from build123d import *

# Parameters (mm, degrees)
BASE_FLANGE1_DEPTH           = 2.65684
EDGE_FLANGE1_DEPTH           = 254
EDGE_FLANGE2_STRIP_W         = 16.97736
EDGE_FLANGE2_STRIP_H         = 2.65684
EDGE_FLANGE2_STRIP_CUT_DEPTH = 112.395
EDGE_FLANGE2_DEPTH           = 112.395
EDGE_FLANGE3_DEPTH           = 112.395
EDGE_FLANGE4_DEPTH           = 248.16816
SKETCH22_R                   = 6.35
CUT_EXTRUDE1_DEPTH           = 2.65684
SKETCH23_R                   = 6.35
CUT_EXTRUDE2_DEPTH           = 2.65684
SKETCH24_R                   = 6.35
CUT_EXTRUDE3_DEPTH           = 2.65684


# Sheet-metal steps are written as plain solids
with BuildPart() as part:
    # Sketch1 → Base-Flange1 (new body)
    with BuildSketch(Plane.XY):
        with BuildLine():
            Line((0, 0), (355.6, 0))
            Line((355.6, 0), (355.6, 254))
            Line((355.6, 254), (193.04, 254))
            ThreePointArc((193.04, 254), (177.8, 238.76), (162.56, 254))
            Line((162.56, 254), (0, 254))
            Line((0, 254), (0, 0))
        make_face()
    extrude(amount=-BASE_FLANGE1_DEPTH)

    # Edge-Flange1 section (across the edge) → Edge-Flange1 (add)
    with BuildSketch(Plane(origin=(-3.175, 0, -2.65684), x_dir=(1, 0, 0), z_dir=(0, 1, 0))):
        with BuildLine():
            Line((-2.65684, 3.175), (-2.65684, 115.57))
            Line((-2.65684, 115.57), (0, 115.57))
            Line((0, 115.57), (0, 3.175))
            ThreePointArc((0, 3.175), (0.92993597, 0.92993597), (3.175, 0))
            Line((3.175, 0), (3.175, -2.65684))
            ThreePointArc((3.175, -2.65684), (-0.948733611, -0.948733611), (-2.65684, 3.175))
        make_face()
    extrude(amount=EDGE_FLANGE1_DEPTH)

    # Edge-Flange2 strip (across the edge) → Edge-Flange2 strip cut (cut)
    with BuildSketch(Plane(origin=(-5.83184, 254, -5.83184), x_dir=(0, -1, 0), z_dir=(0, 0, -1))):
        with Locations((-2.65684, -1.32842)):
            Rectangle(EDGE_FLANGE2_STRIP_W, EDGE_FLANGE2_STRIP_H)
    extrude(amount=EDGE_FLANGE2_STRIP_CUT_DEPTH, mode=Mode.SUBTRACT)

    # Edge-Flange2 section (across the edge) → Edge-Flange2 (add)
    with BuildSketch(Plane(origin=(-5.83184, 254, -5.83184), x_dir=(0, -1, 0), z_dir=(0, 0, -1))):
        with BuildLine():
            Line((0, 3.175), (0, 57.15))
            Line((0, 57.15), (2.65684, 57.15))
            Line((2.65684, 57.15), (2.65684, 3.175))
            ThreePointArc((2.65684, 3.175), (3.58677597, 0.92993597), (5.83184, 0))
            Line((5.83184, 0), (5.83184, -2.65684))
            ThreePointArc((5.83184, -2.65684), (1.708106389, -0.948733611), (0, 3.175))
        make_face()
    extrude(amount=EDGE_FLANGE2_DEPTH)

    # Edge-Flange3 section (across the edge) → Edge-Flange3 (add)
    with BuildSketch(Plane(origin=(-5.83184, -3.175, -118.22684), x_dir=(0, 1, 0), z_dir=(0, 0, 1))):
        with BuildLine():
            Line((-2.65684, 3.175), (-2.65684, 57.15))
            Line((-2.65684, 57.15), (0, 57.15))
            Line((0, 57.15), (0, 3.175))
            ThreePointArc((0, 3.175), (0.92993597, 0.92993597), (3.175, 0))
            Line((3.175, 0), (3.175, -2.65684))
            ThreePointArc((3.175, -2.65684), (-0.948733611, -0.948733611), (-2.65684, 3.175))
        make_face()
    extrude(amount=EDGE_FLANGE3_DEPTH)

    # Edge-Flange4 section (across the edge) → Edge-Flange4 (add)
    with BuildSketch(Plane(origin=(-3.175, 0, -121.40184), x_dir=(0, 0, 1), z_dir=(0, 1, 0))):
        with BuildLine():
            Line((-2.65684, 3.175), (-2.65684, 25.4))
            Line((-2.65684, 25.4), (0, 25.4))
            Line((0, 25.4), (0, 3.175))
            ThreePointArc((0, 3.175), (0.92993597, 0.92993597), (3.175, 0))
            Line((3.175, 0), (3.175, -2.65684))
            ThreePointArc((3.175, -2.65684), (-0.948733611, -0.948733611), (-2.65684, 3.175))
        make_face()
    extrude(amount=EDGE_FLANGE4_DEPTH)

    # Sketch22 → Cut-Extrude1 (cut)
    with BuildSketch(Plane(origin=(0, 254, 0), x_dir=(1, 0, 0), z_dir=(0, 1, 0))):
        with Locations(Location((-40.76446, 86.995, 0), (0, 0, 180))):
            Circle(SKETCH22_R)
        with Locations(Location((-40.76446, 36.195, 0), (0, 0, 180))):
            Circle(SKETCH22_R)
    extrude(amount=-CUT_EXTRUDE1_DEPTH, mode=Mode.SUBTRACT)

    # Sketch23 → Cut-Extrude2 (cut)
    with BuildSketch(Plane(origin=(0, -3.175, 0), x_dir=(1, 0, 0), z_dir=(0, 1, 0))):
        with Locations(Location((-34.40684, 86.36, 0), (0, 0, 180))):
            Circle(SKETCH23_R)
        with Locations(Location((-34.40684, 35.56, 0), (0, 0, 180))):
            Circle(SKETCH23_R)
    extrude(amount=-CUT_EXTRUDE2_DEPTH, mode=Mode.SUBTRACT)

    # Sketch24 → Cut-Extrude3 (cut)
    with BuildSketch(Plane.ZY.offset(5.83184)):
        with Locations((-86.995, 41.79316)):
            Circle(SKETCH24_R)
        with Locations((-34.40684, 41.79316)):
            Circle(SKETCH24_R)
    extrude(amount=-CUT_EXTRUDE3_DEPTH, mode=Mode.SUBTRACT)


solid = part.part
For this review, take the finished solid that the model builds, in its own axes (mm). A direction names the side the tool comes from. Round coordinates to 2 decimals unless told otherwise and drop trailing zeros. Write each loop counter-clockwise with the first axis right and the second up, starting at its lowest first coordinate (ties: lowest second). Pieces come first, ordered by that corner, then holes. Notation, with made-up numbers: (25, 27.25) -> (32, 27.25) arc R15 ccw to (32, 51.25) -> close; hole circle Ø11 at (63, 67.5). An arc over 180 degrees is marked (long way). Put each result on its own line as item: value.
Q1. Consider section B-B on z = -70.5. State the section outline as (x, y) points (3 decimals), and give its area (3 significant figures).
Determined:
outline: (-62.982, -5.832) -> (-9.007, -5.832) arc R5.832 ccw to (-3.175, 0) -> (-3.175, 248.168) arc R5.832 ccw to (-9.007, 254) -> (-62.982, 254) -> (-62.982, 251.343) -> (-9.007, 251.343) arc R3.175 cw to (-5.832, 248.168) -> (-5.832, 0) arc R3.175 cw to (-9.007, -3.175) -> (-62.982, -3.175) -> close
area: 984 mm^2
Q2. Consider section D-D on x = 49. State the section outline as (y, z) points.
Determined:
outline: (0, -2.66) -> (254, -2.66) -> (254, 0) -> (0, 0) -> close
Q3. Consider section A-A on y = 183. State the section outline as (x, z) points (3 decimals).
Determined:
outline: (-5.832, -118.227) arc R5.832 ccw to (0, -124.059) -> (22.225, -124.059) -> (22.225, -121.402) -> (0, -121.402) arc R3.175 cw to (-3.175, -118.227) -> (-3.175, -5.832) arc R3.175 cw to (0, -2.657) -> (355.6, -2.657) -> (355.6, 0) -> (0, 0) arc R5.832 ccw to (-5.832, -5.832) -> close
Q4. The part is to be moulded in two halves that separate along Z. For faces 6 (the cylindrical face through (-4.52, 42.07, -40.75)), 7 (the cylindrical face through (178.135, 238.764, -1.31)), 8 (the flat face through (11, 122, -124.059)), say which applies: released by +Z, released by -Z, zero draft, split by the parting line, or undercut.
Determined:
face 6: undercut
face 7: zero draft
face 8: released by -Z
Q5. Machinability: for faces 1 (the flat face through (-36, -5.832, -63)), 2 (the cylindrical face through (-37.821, -4.485, -81.006)), 3 (the cylindrical face through (-34.42, 252.69, -35.92)), 4 (the flat face through (11, 122, -121.402)), 5 (the flat face through (-36, -3.175, -63)), which of the approach directions +Z, -Z, +X, -X, +Y, -Y give a long, thin tool a straight path to every point of the face, cutting with its end or side? Answer none if there is none.
Determined:
face 1: +Z, -Z, +X, -X, -Y
face 2: -Y
face 3: +Y
face 4: +X, +Y, -Y
face 5: +Z, -Z, -X
Q6. To check wall thickness, follow L1, parallel to Y at x = -38, z = -112 (3 decimals); L2, parallel to Z at x = 189.5, y = 199; L3, parallel to X at y = -4, z = -86. State the ranges of each line that lie inside material, in increasing order. Write a range as [from, to].
Determined:
L1: y = [-5.832, -3.175], [251.343, 254]
L2: z = [-2.66, 0]
L3: x = [-62.98, -40.75], [-28.07, -4.76]
Q7. Clearance check with flat-ended pins moving along their axes: pin 1 Ø12 at (x, y) = (277.5, 195) entering from -Z; pin 2 Ø3 at (y, z) = (137, -61) entering from -X; pin 3 Ø4 at (y, z) = (144, -24) entering from +X (3 decimals); pin 4 Ø10 at (y, z) = (41.79, -87) entering from +X. State where each tip first meets the part, or that it passes through.
Determined:
pin 1: stops at z = -2.66
pin 2: stops at x = -5.83
pin 3: stops at x = -3.175
pin 4: passes through
Q8. Consider section C-C on x = 177.8. State the section outline as (y, z) points, and give its area (3 significant figures).
Determined:
outline: (0, -2.66) -> (238.76, -2.66) -> (238.76, 0) -> (0, 0) -> close
area: 634 mm^2
